Source: CAD feature listing. Evaluate the final solid. Frame: model axes, mm. Face numbers are marked on the shaded views. A direction names the side the tool comes from. Give positions to 0.01 mm unless a question says otherwise; leave off trailing zeros. Loops run counter-clockwise (first coordinate to the right, second up) from the corner with the lowest first, then second, coordinate; pieces in that order, holes last. Notation, with made-up numbers: (-18.5, -28.75) -> (-9.5, -28.75) arc R27 ccw to (-9.5, 9.25) -> close; hole circle Ø10 at (81.25, 67.5). An arc over 180 degrees is marked (long way). Put each result on its own line as item: value.
```python
from build123d import *

# Parameters (mm, degrees)
F0_R     = 2.54
F1_DEPTH = 1.27
F2_R     = 3.9875638358
F3_DEPTH = 1.27
F4_W     = 0.9389580227
F4_H     = 0.7173512131
F5_DEPTH = 2.54
F6_W     = 1.0421685874
F6_H     = 0.7513510063
F7_DEPTH = 0.508


with BuildPart() as f1:
    # F0 (on Right) → F1 (new body)
    with BuildSketch(Plane.YZ):
        with Locations((-2.8381347656, 0.8016005158)):
            Circle(F0_R)
    extrude(amount=F1_DEPTH)

    # F2 (on face) → F3 (join)
    with BuildSketch(Plane.YZ.offset(1.27)):
        with Locations((-2.8381347656, 0.8016005158)):
            Circle(F2_R)
    extrude(amount=F3_DEPTH)

    # F4 (on face) → F5 (join)
    with BuildSketch(Plane(origin=(0, 0, 0), x_dir=(0, -1, 0), z_dir=(-1, 0, 0))):
        with Locations((2.8381347656, 0.8016005158)):
            Rectangle(F4_W, F4_H)
    extrude(amount=F5_DEPTH)

    # F6 (on face) → F7 (cut)
    with BuildSketch(Plane.YZ.offset(2.54)):
        with BuildLine():
            Line((-3.3592190593, 1.177276019), (-2.3170504719, 1.177276019))
            Line((-2.3170504719, 1.177276019), (-2.3170504719, 4.7549707873))
            ThreePointArc((-2.3170504719, 4.7549707873), (-2.8381347656, 4.7891643516), (-3.3592190593, 4.7549707873))
            Line((-3.3592190593, 4.7549707873), (-3.3592190593, 1.177276019))
        make_face()
        with BuildLine():
            Line((-2.3170504719, 1.177276019), (-2.3170504719, 0.4259250127))
            Line((-2.3170504719, 0.4259250127), (1.1316930972, 0.4259250127))
            ThreePointArc((1.1316930972, 0.4259250127), (1.1449926089, 0.613553548), (1.1494290701, 0.8016005158))
            ThreePointArc((1.1494290701, 0.8016005158), (1.1449926089, 0.9896474837), (1.1316930972, 1.177276019))
            Line((1.1316930972, 1.177276019), (-2.3170504719, 1.177276019))
        make_face()
        with BuildLine():
            ThreePointArc((-3.3592190593, -3.1517697556), (-2.8381347656, -3.1859633199), (-2.3170504719, -3.1517697556))
            Line((-2.3170504719, -3.1517697556), (-2.3170504719, 0.4259250127))
            Line((-2.3170504719, 0.4259250127), (-3.3592190593, 0.4259250127))
            Line((-3.3592190593, 0.4259250127), (-3.3592190593, -3.1517697556))
        make_face()
        with BuildLine():
            Line((-6.8079626285, 0.4259250127), (-3.3592190593, 0.4259250127))
            Line((-3.3592190593, 0.4259250127), (-3.3592190593, 1.177276019))
            Line((-3.3592190593, 1.177276019), (-6.8079626285, 1.177276019))
            ThreePointArc((-6.8079626285, 1.177276019), (-6.8256986014, 0.8016005158), (-6.8079626285, 0.4259250127))
        make_face()
        with Locations((-2.8381347656, 0.8016005158)):
            Rectangle(F6_W, F6_H)
    extrude(amount=-F7_DEPTH, mode=Mode.SUBTRACT)


solid = f1.part
```
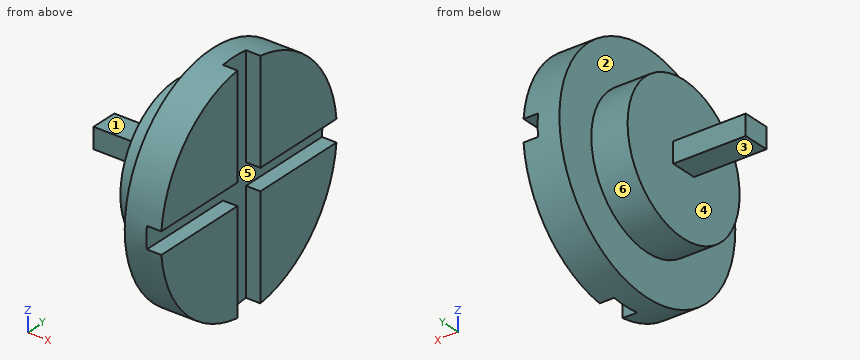
(1) Section A-A on z = -1.25. Return loops of the section in (x, y).
Calculated:
outline: (0, -4.34) -> (1.27, -4.34) -> (1.27, -6.26) -> (2.54, -6.26) -> (2.54, -3.36) -> (2.03, -3.36) -> (2.03, -2.32) -> (2.54, -2.32) -> (2.54, 0.58) -> (1.27, 0.58) -> (1.27, -1.34) -> (0, -1.34) -> close
(2) Line query: probe 1 along X at (y, z) = (0.5, 0.5); probe 2 along X at (y, z) = (-4.5, 0); probe 3 along Z at (x, y) = (-1.75, -3). Output: solid intervals per line, ascending. Write a range as from..to.
Calculated:
probe 1: x = 1.27..2.03
probe 2: x = 0..2.54
probe 3: z = 0.44..1.16
(3) Draft query along Z for the marked faces 4, 5 and 6. Return one class per face: released by +Z, released by -Z, zero draft, split by the parting line, or undercut.
Calculated:
face 4: zero draft
face 5: undercut
face 6: split by the parting line
(4) Section C-C on x = -0.6. Return loops of the section in (y, z), then the cut area to 3 significant figures.
Calculated:
outline: (-3.31, 0.44) -> (-2.37, 0.44) -> (-2.37, 1.16) -> (-3.31, 1.16) -> close
area: 0.674 mm²
(5) Reachability of the marked faces 1, 2 and 3 from +Z, -Z, +X, -X, +Y, -Y: full face, straight path, thin tool, end or side. Return the list, or none.
Calculated:
face 1: +Z, -X, +Y, -Y
face 2: -X
face 3: -Z, -X, +Y, -Y
(6) First-contact query: P1, Ø0.6, axis at x = 2, y = -0.5, coming from the +Z side; P2, Ø2, axis at y = -4, z = -1.5, coming from the -X side; P3, Ø0.6, axis at x = 2, z = -2, coming from the +Y side. Flat tips, straight axial feed; report the tip coordinate or a pass-through.
Calculated:
P1: stops at z = 4.23
P2: stops at x = 0
P3: stops at y = 0.27
(7) Section D-D on z = 0.25. Return loops of the section in (x, y).
Calculated:
outline: (0, -5.32) -> (1.27, -5.32) -> (1.27, -6.79) -> (2.54, -6.79) -> (2.54, -3.36) -> (2.03, -3.36) -> (2.03, -2.32) -> (2.54, -2.32) -> (2.54, 1.11) -> (1.27, 1.11) -> (1.27, -0.36) -> (0, -0.36) -> close
(8) Section B-B on y = 0.25. Return loops of the section in (x, z), then the cut area to 3 significant figures.
Calculated:
outline: (1.27, -1.72) -> (2.54, -1.72) -> (2.54, 0.43) -> (2.03, 0.43) -> (2.03, 1.18) -> (2.54, 1.18) -> (2.54, 3.32) -> (1.27, 3.32) -> close
area: 6.03 mm²
